Verification items for the finished model (mm, model axes). A direction names the side the tool comes from. Give positions to 0.01 mm unless a question says otherwise; leave off trailing zeros. Write each loop counter-clockwise with the first axis right and the second up, starting at its lowest first coordinate (ties: lowest second). Pieces come first, ordered by that corner, then holes.
from build123d import *

# Parameters (mm, degrees)
SKETCH1_W           = 355.6
SKETCH1_H           = 203.2
BOSS_EXTRUDE1_DEPTH = 3.175
BOSS_EXTRUDE2_DEPTH = 6.35


with BuildPart() as part:
    # Sketch1 → Boss-Extrude1 (new body, symmetric)
    with BuildSketch(Plane(origin=(0, 0, 0), x_dir=(1, 0, 0), z_dir=(0, 1, 0))):
        Rectangle(SKETCH1_W, SKETCH1_H)
    extrude(amount=BOSS_EXTRUDE1_DEPTH, both=True)

    # Sketch2 → Boss-Extrude2 (add, symmetric)
    with BuildSketch(Plane.XY):
        Polygon((-101.6, 3.175), (-101.6, 104.775), (101.6, 104.775), (101.6, 3.175), (88.9, 3.175), (88.9, 92.075), (-88.9, 92.075), (-88.9, 3.175), align=None)
    extrude(amount=BOSS_EXTRUDE2_DEPTH, both=True)


solid = part.part
Item 1: Scan lines: line 1 along Y through (x, z) = (36.5, 1) (3 decimals); line 2 along Z through (x, y) = (-97, 30); line 3 along Y through (x, z) = (103.5, 1) (3 decimals). Record each from-to range of solid material in increasing order.
Answer key:
line 1: y = -3.175 to 3.175, 92.075 to 104.775
line 2: z = -6.35 to 6.35
line 3: y = -3.175 to 3.175
Item 2: Sectioned sample at D-D on x = -128.5. Record the cut outline in (y, z) (3 decimals).
Answer key:
outline: (-3.175, -101.6) - (3.175, -101.6) - (3.175, 101.6) - (-3.175, 101.6) - close
Item 3: Depth check by flat-ended pin: pin 1 (6 mm diameter, centred on x = -6.5, z = -13, fed in from +Y) (3 decimals); pin 2 (1 mm diameter, centred on y = 40, z = 0, fed in from -X); pin 3 (6.5 mm diameter, centred on y = 54, z = 1, fed in from +X). Enter the tip coordinate at first touch or a pass-through.
Answer key:
pin 1: stops at y = 3.175
pin 2: stops at x = -101.6
pin 3: stops at x = 101.6
Item 4: Sectioned sample at B-B on x = -71.5. Record the cut outline in (y, z) (3 decimals).
Answer key:
outline: (-3.175, -101.6) - (3.175, -101.6) - (3.175, 101.6) - (-3.175, 101.6) - close; (92.075, -6.35) - (104.775, -6.35) - (104.775, 6.35) - (92.075, 6.35) - close
Item 5: Sectioned sample at C-C on z = 54.5. Record the cut outline in (x, y) (3 decimals), then the cut area to 3 significant figures.
Answer key:
outline: (-177.8, -3.175) - (177.8, -3.175) - (177.8, 3.175) - (-177.8, 3.175) - close
area: 2,260 mm2
Item 6: Set-up check for faces 5 (the face through (0, 96, 6.35)), 6 (the face through (-1, 104.775, 0)), 7 (the face through (-101.6, 53, 0)), 8 (the face through (-2, -3.175, -1)), 9 (the face through (-88.9, 48, 0)): record each of +Z, -Z, +X, -X, +Y, -Y from which the full face is reachable in a straight line by a thin tool's end or side.
Answer key:
face 5: +Z, +X, -X, +Y
face 6: +Z, -Z, +X, -X, +Y
face 7: +Z, -Z, -X, +Y
face 8: +Z, -Z, +X, -X, -Y
face 9: +Z, -Z
Item 7: Sectioned sample at A-A on y = 68. Record the cut outline in (x, z), then the cut area to 3 significant figures.
Answer key:
outline: (-101.6, -6.35) - (-88.9, -6.35) - (-88.9, 6.35) - (-101.6, 6.35) - close; (88.9, -6.35) - (101.6, -6.35) - (101.6, 6.35) - (88.9, 6.35) - close
area: 323 mm2
Item 8: Release check for a two-part mould opening along X. For faces 1 (the face through (101.6, 55, 0)), 2 (the face through (88.9, 47, 0)), 3 (the face through (1, 92.075, 0)), 4 (the face through (0, 96, -6.35)) record: released by +X, released by -X, zero draft, split by the parting line, or undercut.
Answer key:
face 1: released by +X
face 2: undercut
face 3: undercut
face 4: zero draft
